Autodesk Inventor part; units mm, degrees
ref_plane "YZ Plane" through (0, 0, 0) normal (1, 0, 0) x (0, 1, 0)
ref_plane "XZ Plane" through (0, 0, 0) normal (0, 1, 0) x (-1, 0, 0)
ref_plane "XY Plane" through (0, 0, 0) normal (0, 0, 1) x (1, 0, 0)
sketch "Sketch1" plane through (0, 0, 0) normal (0, 1, 0) x (-1, 0, 0)
  line L0 (-15, -41.5) -> (15, -41.5)
  line L1 (15, -41.5) -> (15, 41.5)
  line L2 (15, 41.5) -> (-15, 41.5)
  line L3 (-15, 41.5) -> (-15, -41.5)
  line L4 (-15, -41.5) -> (15, 41.5) construction
  line L5 (15, -41.5) -> (-15, 41.5) construction
  point P0 (0, 0)
  dimension "d0" = 30
  dimension "d1" = 83
extrude "Extrusion1" add sketch "Sketch1" along normal blind 15
sketch "Sketch2" plane through (0, 15, 0) normal (0, 1, 0) x (1, 0, 0)
  line L0 (-15, 41.5) -> (-15, -41.5)
  line L1 (15, 25) -> (-15, 25)
  line L2 (-15, 25) -> (-15, -25)
  line L3 (-15, -25) -> (15, -25)
  line L4 (15, -25) -> (15, 25)
  line L5 (15, 25) -> (-15, -25) construction
  line L6 (-15, 25) -> (15, -25) construction
  point P0 (0, 0)
  point P1 (-15, 25)
  dimension "d4" = 50
extrude "Extrusion2" add sketch "Sketch2" along normal blind 50
chamfer "Chamfer1" distance 10 angle 45 2 edges at (0, 65, 25) (0, 65, -25)
sketch "Sketch3" plane through (0, 15, 0) normal (0, 1, 0) x (1, 0, 0)
  line L0 (-15, 41.5) -> (-15, 25)
  line L1 (15, 41.5) -> (-15, 41.5)
  point P0 (0, 0)
  point P1 (0, 32.5)
  point P2 (-15, 33.25)
  dimension "d10" = 15
  dimension "d11" = 9
hole "Hole1" at (0, 15, -32.5) direction (0, -1, 0) diameter 7.134 end through all
mirror "Mirror1" about plane through (0, 0, 0) normal (0, 0, 1) of "Hole1"
sketch "Sketch4" plane through (-15, 0, -41.5) normal (-1, 0, 0) x (0, 0, 1)
  circle A0 centre (41.5, 40) radius 17.5
  line L0 (26.5, 65) -> (56.5, 65)
  line L1 (66.5, 15) -> (66.5, 55)
  point P0 (41.5, 0)
  dimension "d19" = 35
  dimension "d20" = 25
  dimension "d21" = 25
extrude "Extrusion3" cut sketch "Sketch4" against normal blind 50
properties part number "Pillow_block" material "Brass, Soft Yellow"
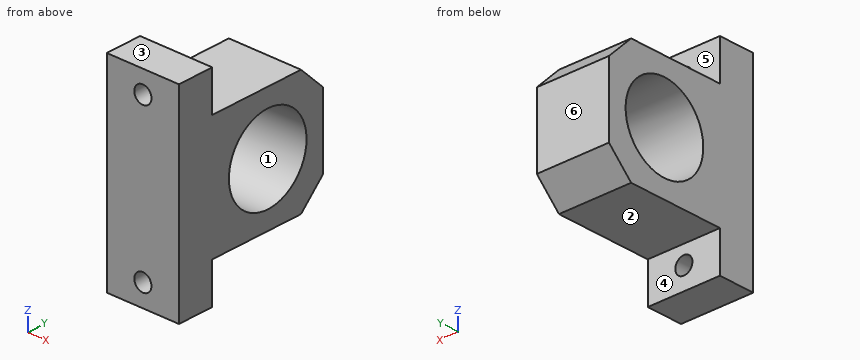
Part model, mm, in its own coordinate system. Face numbers are marked on the shaded views. A direction names the side the tool comes from. Round coordinates to 2 decimals unless told otherwise and drop trailing zeros. Write each loop counter-clockwise with the first axis right and the second up, starting at its lowest first coordinate (ties: lowest second). Pieces come first, ordered by that corner, then holes. Notation, with made-up numbers: M -15.5,18 L 19.5,18 A19 ccw 19.5,38 Z; hole C 56,-23.5 d7. An arc over 180 degrees is marked long. Answer as CSV lines item,"result". Start each with the question number.
1) Band-saw the part on C-C (x = 0). List the corners of the cut face in (y, z).
2) Mould opens along Z. For the marked faces 1, 2 and 3 say: +Z half, -Z half, draft (parallel to the pull), parting line (faces both ways), or undercut.
3) Band-saw the part on D-D (x = -9). List the corners of the cut face in (y, z), then the cut area to 3 significant figures.
4) Drill centre lines: L1, parallel to Z at x = 0, y = 6.75; L2, parallel to X at y = 3, z = -32.5; L3, parallel to Y at x = 9, z = 0. Where is each one in solid material? Low to high.
5) Drop flat-ended pins along their axis: pin 1 (15 mm diameter, centred on x = 0, y = 36, fed in from +Z); pin 2 (4.5 mm diameter, centred on x = 0, z = 32.5, fed in from -Y) (1 decimal); pin 3 (3 mm diameter, centred on x = 6.5, y = 32.5, fed in from -Z); pin 4 (8 mm diameter, centred on x = 3.5, z = -35.5, fed in from +Y). Give the stop position or say it passes through.
6) Band-saw the part on B-B (y = 40). List the corners of the cut face in (x, z).
7) Band-saw the part on A-A (z = 0). List the corners of the cut face in (x, y), then the cut area to 3 significant figures.
8) Which spindle directions (+Z, -Z, +X, -X, +Y, -Y) get a long thin tool onto all of the face, cutting with end or side? Do the marked faces 4, 5 and 6. Say none if no direction does.
Worked out:
1,outline,"M 0,-41.5 L 15,-41.5 L 15,-36.07 L 0,-36.07 Z; M 0,-28.93 L 15,-28.93 L 15,-25 L 55,-25 L 65,-15 L 65,15 L 55,25 L 15,25 L 15,28.93 L 0,28.93 Z; M 0,36.07 L 15,36.07 L 15,41.5 L 0,41.5 Z; hole C 40,0 d35"
2,face 1,"undercut"
2,face 2,"-Z half"
2,face 3,"+Z half"
3,outline,"M 0,-41.5 L 15,-41.5 L 15,-25 L 55,-25 L 65,-15 L 65,15 L 55,25 L 15,25 L 15,41.5 L 0,41.5 Z; hole C 40,0 d35"
3,area,"2,680 mm²"
4,L1,"-41.5 to -36.07, -28.93 to 28.93, 36.07 to 41.5"
4,L2,"-15 to -3.57, 3.57 to 15"
4,L3,"0 to 22.5, 57.5 to 65"
5,pin 1,"z = 25"
5,pin 2,"through"
5,pin 3,"z = -25"
5,pin 4,"y = 15"
6,outline,"M -15,-25 L 15,-25 L 15,-17.5 L -15,-17.5 Z; M -15,17.5 L 15,17.5 L 15,25 L -15,25 Z"
7,outline,"M -15,0 L 15,0 L 15,22.5 L -15,22.5 Z; M -15,57.5 L 15,57.5 L 15,65 L -15,65 Z"
7,area,"900 mm²"
8,face 4,"-Z, +X, -X, +Y"
8,face 5,"+Z, +X, -X, +Y"
8,face 6,"+Z, -Z, +X, -X, +Y"
